Geometry check sheet. Reference: drawing and pictorial views, mm from the part's lowest x, y, z. A direction names the side the tool comes from. Give positions to 0.01 mm unless a question says otherwise; leave off trailing zeros. Write each loop counter-clockwise with the first axis right and the second up, starting at its lowest first coordinate (ties: lowest second). Pieces come first, ordered by that corner, then holes. Notation, with made-up numbers: (80, -37.5) - (108, -37.5) arc R35 ccw to (108, -3.5) - close; hole circle Ø8 at (6, 12.5). An arc over 180 degrees is marked (long way). Write item = value, one per line. Start each with the question number.
(1) Thickness scan on L1, parallel to X at y = 15.5, z = 10.5; L2, parallel to X at y = 22.5, z = 13.5; L3, parallel to Z at x = 51.5, y = 19. Record the ranges inside material, lowest first.
(2) Section check B-B, the plane y = 18.5. Enter the section's corners in (x, z).
(3) Section check A-A, the plane z = 18.5. Enter the section's corners in (x, y).
(4) Section check D-D, the plane y = 24. Enter the section's corners in (x, z), plus the area to 3 significant figures.
(5) Access from +Z, -Z, +X, -X, +Y, -Y to the whole of each face (thin tool, end or side, straight path). Record for the marked faces 1 and 2.
(6) Section check C-C, the plane x = 43. Enter the section's corners in (y, z).
(7) Depth check by flat-ended pin: pin 1 Ø1 at (x, z) = (6, 18) entering from +Y; pin 2 Ø6 at (x, y) = (12, 17) entering from -Z; pin 3 Ø2 at (y, z) = (15.5, 24) entering from -X; pin 4 Ø6 at (x, y) = (22.5, 14) entering from +Z. Enter the tip coordinate at first touch or a pass-through.
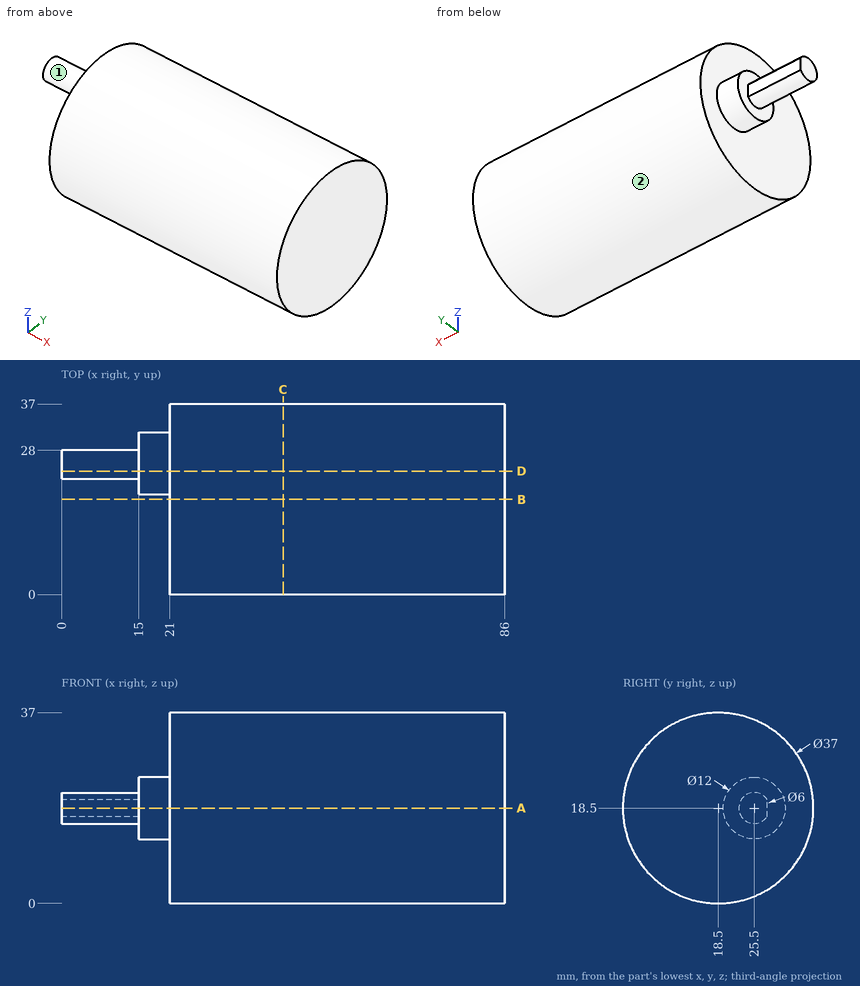
Model answer:
q1.L1 = 21 to 86
q1.L2 = 15 to 86
q1.L3 = 0.01 to 36.99
q2.outline = (21, 0) - (86, 0) - (86, 37) - (21, 37) - close
q3.outline = (0, 22.5) - (15, 22.5) - (15, 19.5) - (21, 19.5) - (21, 0) - (86, 0) - (86, 37) - (21, 37) - (21, 31.5) - (15, 31.5) - (15, 28) - (0, 28) - close
q4.outline = (0, 15.9) - (15, 15.9) - (15, 12.69) - (21, 12.69) - (21, 0.84) - (86, 0.84) - (86, 36.16) - (21, 36.16) - (21, 24.31) - (15, 24.31) - (15, 21.1) - (0, 21.1) - close
q4.area = 2,440 mm²
q5.face_1 = -X
q5.face_2 = +X, -X
q6.outline = circle Ø37 at (18.5, 18.5)
q7.pin_1 = 28
q7.pin_2 = through
q7.pin_3 = 21
q7.pin_4 = 36.94
